Work out the finished part from the listing and answer in its coordinate system (mm). A direction names the side the tool comes from. Round coordinates to 2 decimals unless told otherwise and drop trailing zeros. Loops run counter-clockwise (first coordinate to the right, second up) from the corner with the lowest first, then second, coordinate; pieces in that order, holes last. Notation, with made-up numbers: (-31.5, 85.25) - (13.5, 85.25) arc R15 cw to (13.5, 97.25) - close; hole circle Ø1 at (-22.75, 73). An arc over 180 degrees is marked (long way). Use CSV: the item, a comma, the result in double quotes. Start each with the question number.
from build123d import *

# Parameters (mm, degrees)
BOSS_EXTRUDE1_DEPTH      = 80
BOSS_EXTRUDE1_DEPTH_BACK = 2
SKETCH1_R                = 12.5
CUT_EXTRUDE1_START       = -2
CUT_EXTRUDE1_DEPTH       = 20
SKETCH4_W                = 1.3
SKETCH4_H                = 0.55
SKETCH5_W                = 1.3
SKETCH5_H                = 0.55


with BuildPart() as part:
    # Sketch1 → Boss-Extrude1 (new, two sides: drawn at the far end of the back side and taken through both)
    with BuildSketch(Plane.XY.offset(-BOSS_EXTRUDE1_DEPTH_BACK)):
        Circle(SKETCH1_R)
    extrude(amount=BOSS_EXTRUDE1_DEPTH + BOSS_EXTRUDE1_DEPTH_BACK)

    # Sketch2 → Cut-Extrude1 (cut)
    with BuildSketch(Plane(origin=(0, 0, -2), x_dir=(-1, 0, 0), z_dir=(0, 0, -1)).offset(CUT_EXTRUDE1_START)):
        with BuildLine():
            Line((-4, 11.842719282), (-4, 8.5))
            Line((-4, 8.5), (4, 8.5))
            Line((4, 8.5), (4, 11.842719282))
            ThreePointArc((4, 11.842719282), (0, 12.5), (-4, 11.842719282))
        make_face()
    extrude(amount=-CUT_EXTRUDE1_DEPTH, mode=Mode.SUBTRACT)

    # Sketch4 → Cut-Revolve1 (revolve, cut)
    with BuildSketch(Plane(origin=(0, 0, 0), x_dir=(0, 0, -1), z_dir=(1, 0, 0)), mode=Mode.PRIVATE) as cut_revolve1_sk:
        with Locations((0.65, 12.225)):
            Rectangle(SKETCH4_W, SKETCH4_H)
    revolve(cut_revolve1_sk.sketch.rotate(Axis((0, 0, -5.566261423), (0, 0, 1)), 270), axis=Axis((0, 0, -5.566261423), (0, 0, 1)), mode=Mode.SUBTRACT)

    # Sketch5 → Cut-Revolve2 (revolve, cut)
    with BuildSketch(Plane(origin=(0, 0, 0), x_dir=(0, 0, -1), z_dir=(1, 0, 0)), mode=Mode.PRIVATE) as cut_revolve2_sk:
        with Locations((-20.65, 12.225)):
            Rectangle(SKETCH5_W, SKETCH5_H)
    revolve(cut_revolve2_sk.sketch.rotate(Axis((0, 0, 0), (0, 0, 1)), 90), axis=Axis((0, 0, 0), (0, 0, 1)), mode=Mode.SUBTRACT)


solid = part.part
Item 1: Each of these flat-tipped pins is pushed along its axis until it touches: pin 1 Ø1.7 at (y, z) = (11, 12) entering from -X; pin 2 Ø2 at (x, z) = (-7, 28.5) entering from -Y; pin 3 Ø2 at (x, z) = (-3, 65) entering from -Y. Where does it stop, or does it pass through?
Item 2: Find the intervals of material crossed by probe 1 along Y at (x, z) = (0.5, 7.5); probe 2 along X at (y, z) = (-0.5, 36); probe 3 along Y at (x, z) = (-5.5, 41), in increasing order. Write a range as [from, to].
Item 3: The mould has two halves that part along Z. Classify faces 4 (the flat face through (0, 0, 80)), 5 (the flat face through (-4, 10, 10)), 6 (the flat face through (0, 0, -2)), 7 (the cylindrical face through (11.923, 3.755, -1.655)): pulls with the +Z half, pulls with the -Z half, needs draft (parallel to the pull), parting line crosses it, or undercut.
Item 4: A cutting plane is placed at D-D (y = -10.5). Determine the outline of the cut face in (x, z).
Item 5: A cutting plane is placed at C-C (z = 74.5). Determine the outline of the cut face in (x, y).
Item 6: A cutting plane is placed at B-B (y = 10.25). Determine the outline of the cut face in (x, z).
Item 7: Which of the six approach directions +Z, -Z, +X, -X, +Y, -Y give full straight-line access (tool end or side, diameter ignored) to faces 1 (the cylindrical face through (11.923, 3.755, 50.239)), 2 (the cylindrical face through (-1.556, 11.848, -0.659)), 3 (the flat face through (4, 10, 10))?
Item 8: A cutting plane is placed at A-A (x = 0). Determine the outline of the cut face in (y, z), plus the area to 3 significant figures.
Result sheet:
1,pin 1,"x = -7.3"
1,pin 2,"y = -10.97"
1,pin 3,"y = -12.34"
2,probe 1,"[-12.49, 8.5]"
2,probe 2,"[-12.49, 12.49]"
2,probe 3,"[-11.22, 11.22]"
3,face 4,"pulls with the +Z half"
3,face 5,"undercut"
3,face 6,"pulls with the -Z half"
3,face 7,"needs draft"
4,outline,"(-6.78, -2) - (6.78, -2) - (6.78, -1.3) - (5.71, -1.3) - (5.71, 0) - (6.78, 0) - (6.78, 20) - (5.71, 20) - (5.71, 21.3) - (6.78, 21.3) - (6.78, 80) - (-6.78, 80) - (-6.78, 21.3) - (-5.71, 21.3) - (-5.71, 20) - (-6.78, 20) - (-6.78, 0) - (-5.71, 0) - (-5.71, -1.3) - (-6.78, -1.3) - close"
5,outline,"circle Ø25 at (0, 0)"
6,outline,"(-7.15, -2) - (7.15, -2) - (7.15, -1.3) - (6.14, -1.3) - (6.14, 0) - (7.15, 0) - (7.15, 20) - (6.14, 20) - (6.14, 21.3) - (7.15, 21.3) - (7.15, 80) - (-7.15, 80) - (-7.15, 21.3) - (-6.14, 21.3) - (-6.14, 20) - (-7.15, 20) - (-7.15, 0) - (-6.14, 0) - (-6.14, -1.3) - (-7.15, -1.3) - close; hole (-4, 0) - (4, 0) - (4, 20) - (-4, 20) - close"
7,face 1,"+Z, -Z"
7,face 2,"none"
7,face 3,"+Y"
8,outline,"(-12.5, -2) - (12.5, -2) - (12.5, -1.3) - (11.95, -1.3) - (11.95, 0) - (8.5, 0) - (8.5, 20) - (11.95, 20) - (11.95, 21.3) - (12.5, 21.3) - (12.5, 80) - (-12.5, 80) - (-12.5, 21.3) - (-11.95, 21.3) - (-11.95, 20) - (-12.5, 20) - (-12.5, 0) - (-11.95, 0) - (-11.95, -1.3) - (-12.5, -1.3) - close"
8,area,"1,970 mm^2"
